Check sheet for the drawn part. Datum: minimum x, y, z corner. Units: mm. Coordinates: 2 decimals unless noted, no trailing zeros. Write each loop counter-clockwise with the first axis right and the second up, starting at its lowest first coordinate (ties: lowest second). Pieces come first, ordered by that corner, then holes. Notation, with made-up numbers: M 56.25,15.5 L 68.25,15.5 A14 cw 68.25,32.5 Z; hole C 61.5,69.5 d8. An arc over 180 degrees is marked long. Answer as CSV lines item,"result". Start each with the question number.
Q1. Thickness scan on line 1 along X through (y, z) = (2.6, 23.5); line 2 along Y through (x, z) = (27.5, 25). Record the ranges inside material, lowest first. Write a range as from..to.
Q2. Sectioned sample at B-B, the plane x = 9.5. Record the cut outline in (y, z), then the cut area to 3 significant figures.
Q3. Sectioned sample at C-C, the plane z = 4.5. Record the cut outline in (x, y).
Q4. Sectioned sample at A-A, the plane y = 2.8. Count the separate pieces of the cut face and the enclosed holes in it, then the cut area to 3 significant figures.
Q5. Depth check by flat-ended pin: pin 1 Ø13.5 at (x, z) = (13, 16) entering from +Y. Enter the tip coordinate at first touch or a pass-through.
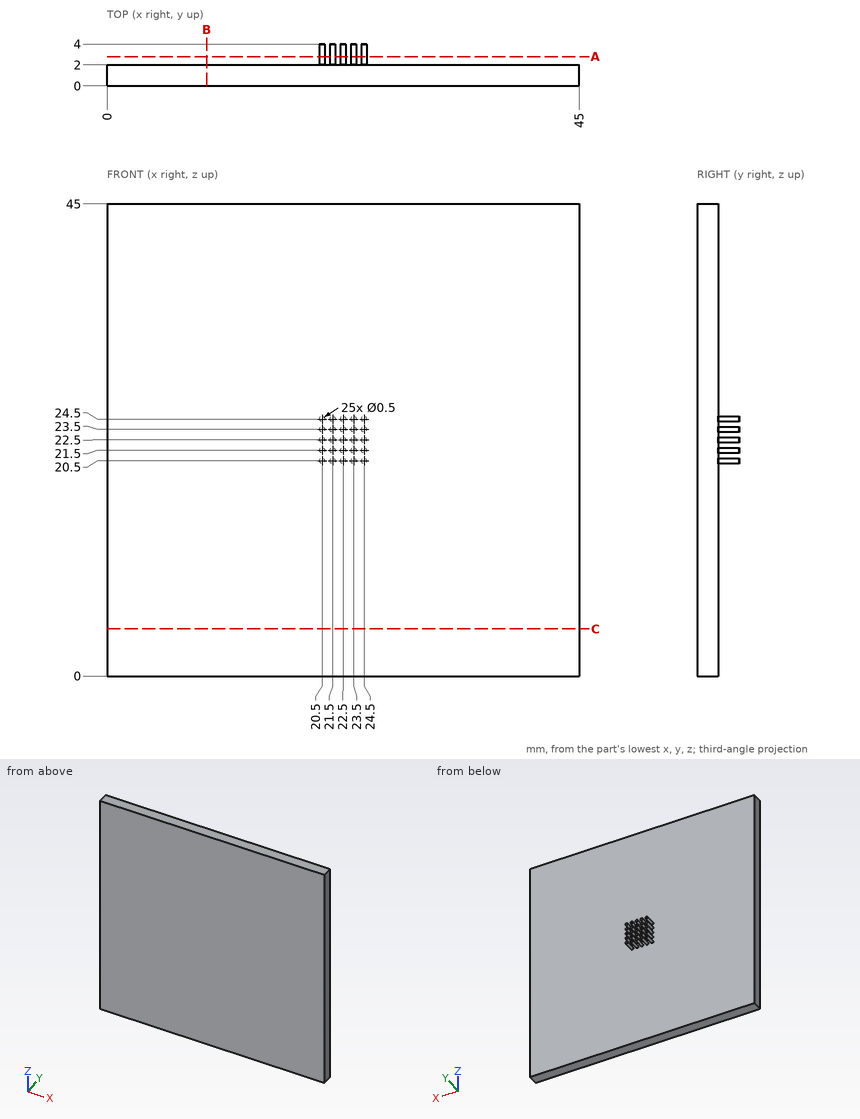
Output:
1,line 1,"x = 20.25..20.75, 21.25..21.75, 22.25..22.75, 23.25..23.75, 24.25..24.75"
1,line 2,"y = 0..2"
2,outline,"M 0,0 L 2,0 L 2,45 L 0,45 Z"
2,area,"90.0 mm^2"
3,outline,"M 0,0 L 45,0 L 45,2 L 0,2 Z"
4,separate pieces,"25"
4,enclosed holes,"0"
4,area,"4.91 mm^2"
5,pin 1,"stops at y = 2"
